Verification items for the finished model (mm, model axes). A direction names the side the tool comes from. Round coordinates to 2 decimals unless told otherwise and drop trailing zeros. Write each loop counter-clockwise with the first axis right and the second up, starting at its lowest first coordinate (ties: lowest second). Pieces come first, ordered by that corner, then holes. Notation, with made-up numbers: M -39,-7.5 L 17,-7.5 A13 ccw 17,-3.5 Z; hole C 67,87 d2. An arc over 180 degrees is marked long. One line per question, with ' | ' between items.
Autodesk Inventor part; units mm, degrees
ref_plane "YZ Plane" through (0, 0, 0) normal (1, 0, 0) x (0, 1, 0)
ref_plane "XZ Plane" through (0, 0, 0) normal (0, 1, 0) x (-1, 0, 0)
ref_plane "XY Plane" through (0, 0, 0) normal (0, 0, 1) x (1, 0, 0)
sketch "Sketch3" plane through (0, 0, 0) normal (1, 0, 0) x (0, 1, 0)
  circle A0 centre (0, 0) radius 12.7
  circle A1 centre (0, 0) radius 50.8
  circle A2 centre (0, 0) radius 101.6
  circle A3 centre (0, 0) radius 44.45
  circle A4 centre (0, 0) radius 9.525
  circle A5 centre (0, 0) radius 6.35
  dimension "d10" = 25.4
  dimension "d11" = 101.6
  dimension "d12" = 203.2
  dimension "d13" = 88.9
  dimension "d14" = 19.05
  dimension "d15" = 12.7
extrude "Extrusion4" add sketch "Sketch3" along normal mid plane 49.53 contours A0 | A1
extrude "Extrusion5" add sketch "Sketch3" along normal mid plane 12.7 contours A3
extrude "Extrusion6" add sketch "Sketch3" along normal mid plane 48.26 contours A2
extrude "Extrusion7" add sketch "Sketch3" along normal mid plane 50.8 contours A4
fillet "Fillet1" radius 12.7 2 edges at (24.13, -101.6, 0) (-24.13, -101.6, 0)
properties part number "wheel"
1. Go/stop test with flat-tipped pins: P1, Ø3, axis at x = -12, y = 34, coming from the +Z side; P2, Ø6, axis at x = 7.5, z = 33, coming from the -Y side; P3, Ø4, axis at x = -11, y = -39, coming from the +Z side. Record where each tip stops, or that it passes through.
Results:
P1: stops at z = 96.25 | P2: stops at y = -97.07 | P3: stops at z = 94.62
2. Thickness scan on line 1 (Z direction, x = 11, y = 0); line 2 (Z direction, x = -10, y = 31.5); line 3 (Y direction, x = -18, z = 8). Record the ranges inside material, lowest first.
Results:
line 1: z = -101.6 to -44.45, -12.7 to -6.35, 6.35 to 12.7, 44.45 to 101.6 | line 2: z = -96.59 to -31.36, 31.36 to 96.59 | line 3: y = -99.45 to -43.72, -9.86 to 9.86, 43.72 to 99.45
3. Mould release check, pull along Y, two halves, no side actions. Record for faces 1 (the face through (-25.4, 6.2, -2)), 2 (the face through (-15.43, -2.75, -12.4)), 3 (the face through (-25.078, -7.559, -5.796)): pulls with the +Y half, pulls with the -Y half, needs draft (parallel to the pull), parting line crosses it, or undercut.
Results:
face 1: needs draft | face 2: undercut | face 3: parting line crosses it
4. Tool access check on faces 4 (the face through (-15.429, 42.397, 13.352)), 5 (the face through (15.43, -2.75, 12.4)), 6 (the face through (25.4, 6.2, -2)). Record the directions out of +Z, -Z, +X, -X, +Y, -Y that give a thin tool (end or side, any length) a straight path to the whole face; none if there is none.
Results:
face 4: -X | face 5: +X | face 6: +Z, -Z, +X, +Y, -Y
5. Section check A-A, the plane x = 20.5. Record the cut outline in (y, z), then the cut area to 3 significant figures.
Results:
outline: C 0,0 d195.58; C 0,0 d25.4; hole C 0,0 d88.9; hole C 0,0 d12.7 | area: 24,200 mm2
